```python
from build123d import *

# Parameters (mm, degrees)
BOSS_EXTRUDE1_DEPTH        = 26
BOSS_EXTRUDE2_DEPTH        = 15
SKETCH3_W                  = 1
SKETCH3_H                  = 1
BOSS_EXTRUDE3_DEPTH        = 8
CHAMFER1_SIZE              = 0.75
LPATTERN1_COUNT            = 15
LPATTERN1_PITCH            = 2
CHAMFER1_OF_LPATTERN1_SIZE = 0.75
SKETCH5_W                  = 1
SKETCH5_H                  = 1
BOSS_EXTRUDE4_DEPTH        = 8
CHAMFER2_SIZE              = 0.75
LPATTERN2_COUNT            = 15
LPATTERN2_PITCH            = 2
CHAMFER2_OF_LPATTERN2_SIZE = 0.75
SKETCH6_R                  = 2.1
CUT_EXTRUDE1_DEPTH         = 30
SKETCH7_R                  = 3.75
SKETCH7_R_2                = 3.5
CUT_EXTRUDE2_DEPTH         = 7


with BuildPart() as part:
    # Sketch1 → Boss-Extrude1 (new body, symmetric)
    with BuildSketch(Plane(origin=(0, 0, 0), x_dir=(1, 0, 0), z_dir=(0, 1, 0))):
        Polygon((0, 0), (14, 0), (14, -18), (1.75, -18), (0, -16), align=None)
    extrude(amount=BOSS_EXTRUDE1_DEPTH, both=True)

    # Sketch2 → Boss-Extrude2 (add, symmetric)
    with BuildSketch(Plane(origin=(0, 0, 0), x_dir=(1, 0, 0), z_dir=(0, 1, 0))):
        Polygon((14, -18), (14, -33.5), (2, -33.5), (2, -29.25), (10, -29.25), (10, -27.25), (3.5, -27.25), (2, -25.75), (2, -24.25), (10, -24.25), (10, -22.5), (3.5, -22.5), (2, -21), (2, -18), align=None)
    extrude(amount=BOSS_EXTRUDE2_DEPTH, both=True)

    # Sketch3 → Boss-Extrude3 (add)
    with BuildSketch(Plane.ZY.offset(-10)):
        with Locations((28.75, 14.5)):
            Rectangle(SKETCH3_W, SKETCH3_H)
    boss_extrude3 = extrude(amount=BOSS_EXTRUDE3_DEPTH)

    # Chamfer1
    chamfer1_edges = [part.edges().sort_by_distance(p)[0] for p in [
        (2, 14.5, 28.25),
    ]]
    chamfer(chamfer1_edges, length=CHAMFER1_SIZE)

    # LPattern1: Boss-Extrude3 ×15
    with Locations(*[(0, -i * LPATTERN1_PITCH, 0) for i in range(1, LPATTERN1_COUNT)]):
        add(boss_extrude3)

    # Chamfer1 of LPattern1
    chamfer1_of_lpattern1_edges = [part.edges().sort_by_distance(p)[0] for p in [
        (2, 12.5, 28.25),
        (2, 10.5, 28.25),
        (2, 8.5, 28.25),
        (2, 6.5, 28.25),
        (2, 4.5, 28.25),
        (2, 2.5, 28.25),
        (2, 0.5, 28.25),
        (2, -1.5, 28.25),
        (2, -3.5, 28.25),
        (2, -5.5, 28.25),
        (2, -7.5, 28.25),
        (2, -9.5, 28.25),
        (2, -11.5, 28.25),
        (2, -13.5, 28.25),
    ]]
    chamfer(chamfer1_of_lpattern1_edges, length=CHAMFER1_OF_LPATTERN1_SIZE)

    # Sketch5 → Boss-Extrude4 (add)
    with BuildSketch(Plane.ZY.offset(-10)):
        with Locations((23.75, -14.5)):
            Rectangle(SKETCH5_W, SKETCH5_H)
    boss_extrude4 = extrude(amount=BOSS_EXTRUDE4_DEPTH)

    # Chamfer2
    chamfer2_edges = [part.edges().sort_by_distance(p)[0] for p in [
        (2, -14.5, 23.25),
    ]]
    chamfer(chamfer2_edges, length=CHAMFER2_SIZE)

    # LPattern2: Boss-Extrude4 ×15
    with Locations(*[(0, i * LPATTERN2_PITCH, 0) for i in range(1, LPATTERN2_COUNT)]):
        add(boss_extrude4)

    # Chamfer2 of LPattern2
    chamfer2_of_lpattern2_edges = [part.edges().sort_by_distance(p)[0] for p in [
        (2, -12.5, 23.25),
        (2, -10.5, 23.25),
        (2, -8.5, 23.25),
        (2, -6.5, 23.25),
        (2, -4.5, 23.25),
        (2, -2.5, 23.25),
        (2, -0.5, 23.25),
        (2, 1.5, 23.25),
        (2, 3.5, 23.25),
        (2, 5.5, 23.25),
        (2, 7.5, 23.25),
        (2, 9.5, 23.25),
        (2, 11.5, 23.25),
        (2, 13.5, 23.25),
    ]]
    chamfer(chamfer2_of_lpattern2_edges, length=CHAMFER2_OF_LPATTERN2_SIZE)

    # Sketch6 → Cut-Extrude1 (cut)
    with BuildSketch(Plane.XY.offset(18)):
        with Locations((7.875, 19.05)):
            Circle(SKETCH6_R)
        with Locations((7.875, -19.05)):
            Circle(SKETCH6_R)
    extrude(amount=-CUT_EXTRUDE1_DEPTH, mode=Mode.SUBTRACT)

    # Sketch7 → Cut-Extrude2 (cut)
    with BuildSketch(Plane.XY.offset(18)):
        with Locations((7.875, 19.05)):
            Circle(SKETCH7_R)
        with Locations((7.875, -19.05)):
            Circle(SKETCH7_R_2)
    extrude(amount=-CUT_EXTRUDE2_DEPTH, mode=Mode.SUBTRACT)


solid = part.part
```
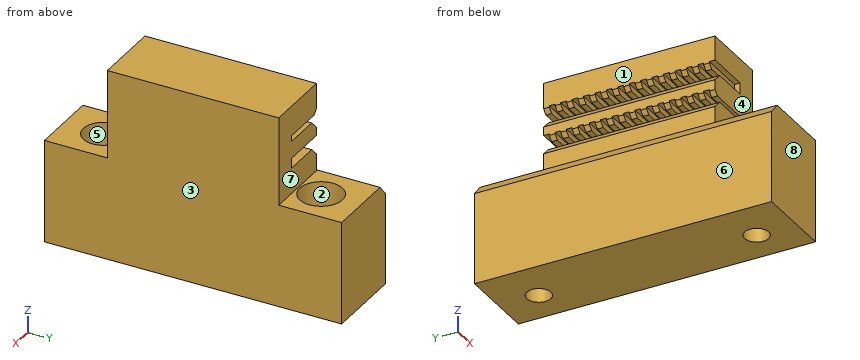
Model file for the job. Use its own axes, mm. Face numbers are marked on the shaded views. A direction names the side the tool comes from. Coordinates: 2 decimals unless noted, no trailing zeros. Order: outer loops, then holes, each group sorted by start corner. A loop starts at its lowest first (then second) coordinate and runs counter-clockwise, first axis right, second up. Notation, with made-up numbers: (-27.5, 47.5) -> (-12.5, 47.5) arc R15 ccw to (-12.5, 76.5) -> close; hole circle Ø1 at (7, 33.5). An arc over 180 degrees is marked (long way). Return JSON: item names as keys, results as strings.
Item 1: Mould opens along Y. For the marked faces 5, 6, 7 and 8 say: pulls with the +Y half, pulls with the -Y half, needs draft (parallel to the pull), parting line crosses it, or undercut.
Model answer:
{"face 5": "undercut", "face 6": "needs draft", "face 7": "pulls with the +Y half", "face 8": "pulls with the -Y half"}
Item 2: Pin check, flat tips, straight feed: P1, Ø0.5, axis at x = 7.5, z = 28.5, coming from the -Y side; P2, Ø1.1, axis at x = 7.5, z = 29, coming from the +Y side; P3, Ø1.1, axis at x = 7.5, z = 23.5, coming from the -Y side. Stop position of each tip, or through.
Model answer:
{"P1": "stops at y = -14", "P2": "stops at y = 15", "P3": "stops at y = -15"}
Item 3: 3-axis set-ups, long thin cutter, end or side, ignore diameter. For the marked faces 1, 2, 3 and 4: which of +Z, -Z, +X, -X, +Y, -Y reach the whole face in a straight line?
Model answer:
{"face 1": "+Z, -X, +Y, -Y", "face 2": "+Z", "face 3": "+Z, -Z, +X, +Y, -Y", "face 4": "+Z, +X, -X, -Y"}
Item 4: Slice it at C-C (x = 12.5). Write the cut outline in (y, z), then the cut area to 3 significant figures.
Model answer:
{"outline": "(-26, 0) -> (26, 0) -> (26, 18) -> (15, 18) -> (15, 33.5) -> (-15, 33.5) -> (-15, 18) -> (-26, 18) -> close", "area": "1,400 mm²"}
Item 5: Slice it at D-D (z = 19). Write the cut outline in (x, y).
Model answer:
{"outline": "(2, -15) -> (14, -15) -> (14, 15) -> (2, 15) -> close"}
Item 6: Slice it at A-A (y = 19.05). Write the cut outline in (x, z) (3 decimals), then the cut area to 3 significant figures.
Model answer:
{"outline": "(0, 0) -> (5.775, 0) -> (5.775, 11) -> (4.125, 11) -> (4.125, 18) -> (1.75, 18) -> (0, 16) -> close; (9.975, 0) -> (14, 0) -> (14, 18) -> (11.625, 18) -> (11.625, 11) -> (9.975, 11) -> close", "area": "152 mm²"}
Item 7: Wall check: line 1 along Z through (x, y) = (9.5, 9.5); line 2 along Z through (x, y) = (9.5, -5.5); line 3 along X through (y, z) = (-19, 15). Give the ranges that are in metal, low to high. Write a range as from..to.
Model answer:
{"line 1": "z = 0..22.5, 23.25..27.25, 29.25..33.5", "line 2": "z = 0..22.5, 24.25..27.25, 28.25..33.5", "line 3": "x = 0..4.38, 11.37..14"}
Item 8: Slice it at B-B (y = -19.05). Write the cut outline in (x, z) (3 decimals).
Model answer:
{"outline": "(0, 0) -> (5.775, 0) -> (5.775, 11) -> (4.375, 11) -> (4.375, 18) -> (1.75, 18) -> (0, 16) -> close; (9.975, 0) -> (14, 0) -> (14, 18) -> (11.375, 18) -> (11.375, 11) -> (9.975, 11) -> close"}
